The listing builds one solid part. Answer for the finished solid, in the listing's coordinates (mm). Coordinates: 2 decimals unless noted, no trailing zeros. Order: outer loops, then holes, each group sorted by start corner. A loop starts at its lowest first (then second) coordinate and runs counter-clockwise, first axis right, second up. Notation, with made-up numbers: (25, 25.25) -> (66, 25.25) arc R26 cw to (66, 61.25) -> close; hole circle Ø10 at (70.5, 18.25). An arc over 180 degrees is marked (long way). Return JSON: item names as keys, results as strings.
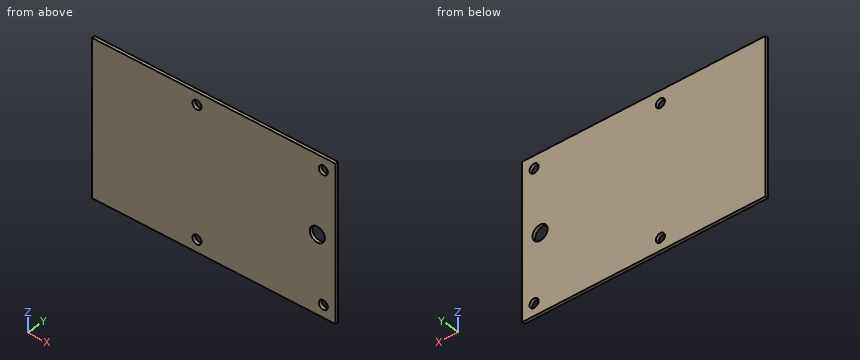
```python
from build123d import *

# Parameters (mm, degrees)
ESBO_O1_W                = 80.9
ESBO_O1_H                = 50
RESSALTO_EXTRUS_O1_DEPTH = 1
ESBO_O2_R                = 1.5
ESBO_O2_R_2              = 2.5
CORTE_EXTRUS_O1_DEPTH    = 48.562616623


with BuildPart() as part:
    # Esboço1 → Ressalto-extrusão1 (new body)
    with BuildSketch(Plane(origin=(0, 0, 0), x_dir=(1, 0, 0), z_dir=(0, 1, 0))):
        Rectangle(ESBO_O1_W, ESBO_O1_H)
    extrude(amount=RESSALTO_EXTRUS_O1_DEPTH)

    # Esboço2 → Corte-extrusão1 (cut, through all)
    with BuildSketch(Plane(origin=(0, 1, 0), x_dir=(1, 0, 0), z_dir=(0, 1, 0))):
        with Locations(Location((36.45, 21, 0), (0, 0, 270))):
            Circle(ESBO_O2_R)
        with Locations(Location((36.45, -21, 0), (0, 0, 270))):
            Circle(ESBO_O2_R)
        with Locations(Location((-5.55, -21, 0), (0, 0, 270))):
            Circle(ESBO_O2_R)
        with Locations(Location((-5.55, 21, 0), (0, 0, 270))):
            Circle(ESBO_O2_R)
        with Locations(Location((34.45, 0, 0), (0, 0, 270))):
            Circle(ESBO_O2_R_2)
    extrude(amount=-CORTE_EXTRUS_O1_DEPTH, mode=Mode.SUBTRACT)


solid = part.part
```
Item 1: Flat-ended cylindrical pins translate along their axes: pin 1 (1.8 mm diameter, centred on x = -5.55, z = -21, fed in from -Y); pin 2 (5 mm diameter, centred on x = 36.45, z = 21, fed in from -Y). Find the tip coordinate at first contact, or state that the pin passes through.
Answer list:
{"pin 1": "through", "pin 2": "y = 0"}
Item 2: The part is cut by section C-C on x = -5.55. Determine the outline of the cut face in (y, z), plus the area to 3 significant figures.
Answer list:
{"outline": "(0, -25) -> (1, -25) -> (1, -22.5) -> (0, -22.5) -> close; (0, -19.5) -> (1, -19.5) -> (1, 19.5) -> (0, 19.5) -> close; (0, 22.5) -> (1, 22.5) -> (1, 25) -> (0, 25) -> close", "area": "44.0 mm2"}
Item 3: The part is cut by section A-A on z = 21. Determine the outline of the cut face in (x, y), plus the area to 3 significant figures.
Answer list:
{"outline": "(-40.45, 0) -> (-7.05, 0) -> (-7.05, 1) -> (-40.45, 1) -> close; (-4.05, 0) -> (34.95, 0) -> (34.95, 1) -> (-4.05, 1) -> close; (37.95, 0) -> (40.45, 0) -> (40.45, 1) -> (37.95, 1) -> close", "area": "74.9 mm2"}
Item 4: The part is cut by section B-B on z = 0. Determine the outline of the cut face in (x, y).
Answer list:
{"outline": "(-40.45, 0) -> (31.95, 0) -> (31.95, 1) -> (-40.45, 1) -> close; (36.95, 0) -> (40.45, 0) -> (40.45, 1) -> (36.95, 1) -> close"}
Item 5: Find the intervals of material crossed by probe 1 along X at (y, z) = (0.7, 21); probe 2 along X at (y, z) = (0.7, 0), in increasing order.
Answer list:
{"probe 1": "-40.45 to -7.05, -4.05 to 34.95, 37.95 to 40.45", "probe 2": "-40.45 to 31.95, 36.95 to 40.45"}
